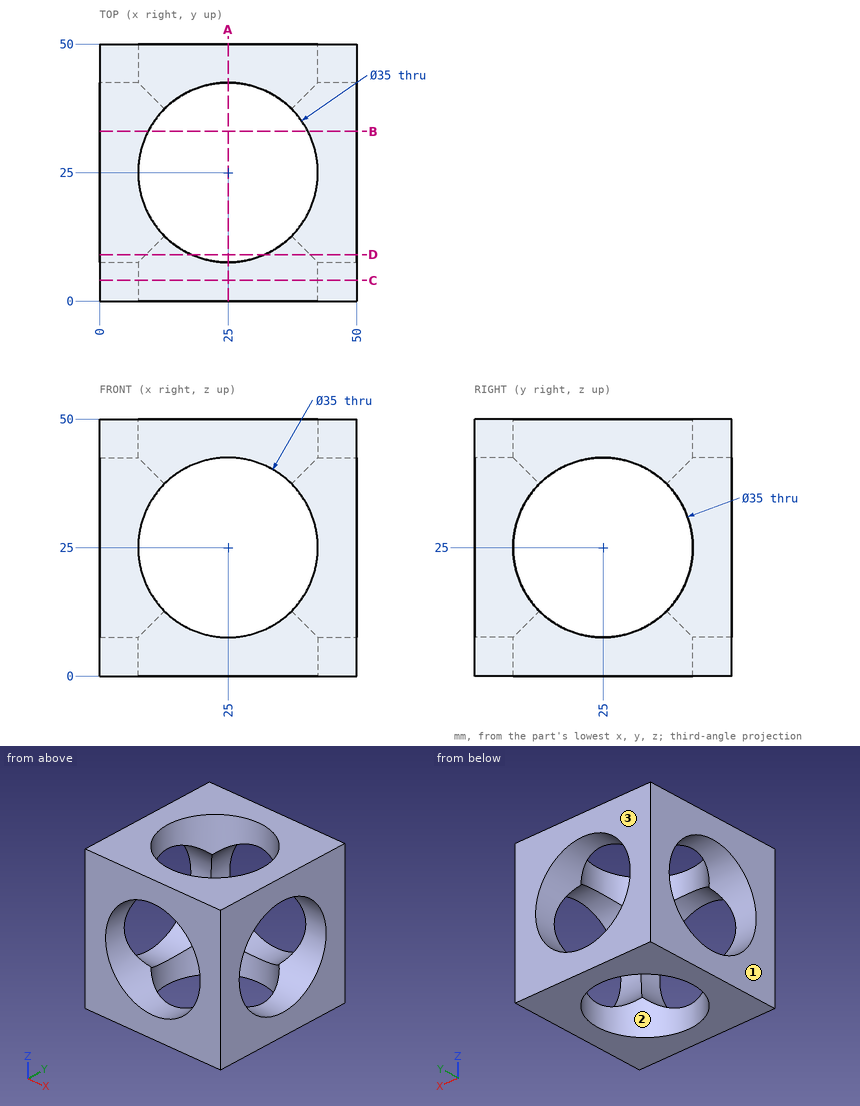
Print and shaded views of the part. All mm, measured from the part's lowest x, y and z. Give positions to 0.01 mm unless a question says otherwise; leave off trailing zeros. Write each loop counter-clockwise with the first axis right and the second up, starting at its lowest first coordinate (ties: lowest second). Pieces come first, ordered by that corner, then holes. Notation, with made-up numbers: (-33.75, -16) -> (16.25, -16) arc R19 cw to (16.25, 7) -> close; hole circle Ø2 at (86, 11). An arc over 180 degrees is marked (long way). Use CSV: the item, a comma, the result in double quotes. Start each with the question number.
1) Cut at B-B on y = 33. List the corners of the cut face in (x, z), plus the area to 3 significant figures.
2) Cut at C-C on y = 4. List the corners of the cut face in (x, z).
3) Two-plate mould, pull along Y, no slides. Class the marked faces 1, 2 and 3: released by +Y, released by -Y, zero draft, split by the parting line, or undercut.
4) Cut at A-A on x = 25. List the corners of the cut face in (y, z).
5) Cut at D-D on y = 9. List the corners of the cut face in (x, z), plus the area to 3 significant figures.
6) Drill centre line: L1, parallel to Z at x = 25, y = 5.75. Where is it in solid material? Low to high.
Final values:
1,outline,"(0, 0) -> (9.44, 0) -> (9.44, 9.44) -> (0, 9.44) -> close; (0, 40.56) -> (9.44, 40.56) -> (9.44, 50) -> (0, 50) -> close; (40.56, 0) -> (50, 0) -> (50, 9.44) -> (40.56, 9.44) -> close; (40.56, 40.56) -> (50, 40.56) -> (50, 50) -> (40.56, 50) -> close"
1,area,"356 mm2"
2,outline,"(0, 0) -> (50, 0) -> (50, 50) -> (0, 50) -> close; hole circle Ø35 at (25, 25)"
3,face 1,"zero draft"
3,face 2,"undercut"
3,face 3,"released by +Y"
4,outline,"(0, 0) -> (7.5, 0) -> (7.5, 7.5) -> (0, 7.5) -> close; (0, 42.5) -> (7.5, 42.5) -> (7.5, 50) -> (0, 50) -> close; (42.5, 0) -> (50, 0) -> (50, 7.5) -> (42.5, 7.5) -> close; (42.5, 42.5) -> (50, 42.5) -> (50, 50) -> (42.5, 50) -> close"
5,outline,"(0, 0) -> (17.91, 0) -> (17.91, 9) arc R17.5 cw to (9, 17.91) -> (0, 17.91) -> close; (0, 32.09) -> (9, 32.09) arc R17.5 cw to (17.91, 41) -> (17.91, 50) -> (0, 50) -> close; (32.09, 0) -> (50, 0) -> (50, 17.91) -> (41, 17.91) arc R17.5 cw to (32.09, 9) -> close; (32.09, 41) arc R17.5 cw to (41, 32.09) -> (50, 32.09) -> (50, 50) -> (32.09, 50) -> close"
5,area,"1,080 mm2"
6,L1,"z = 0 to 7.5, 42.5 to 50"
